from build123d import *

# Parameters (mm, degrees)
ESQUISSE2_W             = 8.320302529
ESQUISSE2_H             = 23.371875391
ESQUISSE2_W_2           = 7.922092332
ENL_V_MAT_EXTRU_1_DEPTH = 32
ENL_V_START             = -2
ENL_V_MAT_EXTRU_2_DEPTH = 2
ESQUISSE4_R             = 1
ENL_V_MAT_EXTRU_3_DEPTH = 4
ESQUISSE5_W             = 12.730996015
ESQUISSE5_H             = 15.162705394
ENL_V_MAT_EXTRU_4_DEPTH = 8


with BuildPart() as part:
    # Esquisse1 → Révolution1 (revolve)
    with BuildSketch(Plane.XY, mode=Mode.PRIVATE) as r_volution1_sk:
        Polygon((-14, 0), (-14, -2), (-3, -2), (-3, -4), (-2, -4), (-2, -7), (0, -7), (0, -11), (14.4, -11), (14.4, -10.25), (46.4, -10.25), (46.4, -3), (48.4, -3), (48.4, 0), align=None)
    revolve(r_volution1_sk.sketch.rotate(Axis((38.703399471, 0, 0), (-1, 0, 0)), 270), axis=Axis((38.703399471, 0, 0), (-1, 0, 0)))

    # Esquisse2 → Enlèv. mat.-Extru.1 (cut)
    with BuildSketch(Plane(origin=(46.4, 0, 0), x_dir=(0, 0, -1), z_dir=(1, 0, 0))):
        with Locations((-11.860151265, -0.490104857)):
            Rectangle(ESQUISSE2_W, ESQUISSE2_H)
        with Locations((11.661046166, -0.490104857)):
            Rectangle(ESQUISSE2_W_2, ESQUISSE2_H)
    extrude(amount=-ENL_V_MAT_EXTRU_1_DEPTH, mode=Mode.SUBTRACT)

    # Esquisse3 → Enlèv. mat.-Extru.2 (cut)
    with BuildSketch(Plane.ZY.offset(2).offset(ENL_V_START)):
        with BuildLine():
            Line((6.792150444, 1.69313093), (1.69313093, 6.792150444))
            ThreePointArc((1.69313093, 6.792150444), (4.949747468, 4.949747468), (6.792150444, 1.69313093))
        make_face()
        with BuildLine():
            Line((-6.792150444, -1.69313093), (-1.69313093, -6.792150444))
            ThreePointArc((-1.69313093, -6.792150444), (-4.949747468, -4.949747468), (-6.792150444, -1.69313093))
        make_face()
    extrude(amount=ENL_V_MAT_EXTRU_2_DEPTH, mode=Mode.SUBTRACT)

    # Esquisse4 → Enlèv. mat.-Extru.3 (cut)
    with BuildSketch(Plane.ZY):
        with Locations((0, 9)):
            Circle(ESQUISSE4_R)
        with Locations((-9, 0)):
            Circle(ESQUISSE4_R)
        with Locations((0, -9)):
            Circle(ESQUISSE4_R)
        with Locations((9, 0)):
            Circle(ESQUISSE4_R)
    extrude(amount=-ENL_V_MAT_EXTRU_3_DEPTH, mode=Mode.SUBTRACT)

    # Esquisse5 → Enlèv. mat.-Extru.4 (cut)
    with BuildSketch(Plane.ZY.offset(14)):
        with Locations((7.865498008, 1.780904513)):
            Rectangle(ESQUISSE5_W, ESQUISSE5_H)
    extrude(amount=-ENL_V_MAT_EXTRU_4_DEPTH, mode=Mode.SUBTRACT)


solid = part.part
Can you work these out from the model? Positions are in its coordinate system, mm. A direction names the side the tool comes from. Give positions to 0.01 mm unless a question says otherwise; leave off trailing zeros. Order: outer loops, then holes, each group sorted by start corner. A loop starts at its lowest first (then second) coordinate and runs counter-clockwise, first axis right, second up. Notation, with made-up numbers: M 12.25,-33.5 L 25.25,-33.5 A19 ccw 25.25,-24.5 Z; hole C -9.5,61 d6. An arc over 180 degrees is marked long. Use a Markdown table: item, result. Add a question column.
Item 1: We'd pull the mould along Z, two halves only. Please class faces 1 (the flat face through (4, 9, 0)), 2 (the flat face through (-14, 0, 0)), 3 (the flat face through (4, -9, 0)), 4 (the cylindrical face through (30.62, 10.25, 0.12)): +Z half, -Z half, draft (parallel to the pull), parting line (faces both ways), or undercut.
Item 2: Suppose I cut it at C-C (x = 44). List the corners of the cut face in (y, z) for me, then the cut area to 3 significant figures.
Item 3: For faces 5 (the flat face through (-0.986, -4.207, -4.278)), 6 (the cylindrical face through (30.62, -10.25, -0.12)), 7 (the flat face through (14.4, 0, -8)), 8 (the flat face through (-10, 0, 1.5)), 9 (the flat face through (4, 0, -9)), which set-ups out of +Z, -Z, +X, -X, +Y, -Y let a thin tool reach every point of the face, with its end or its side?
Item 4: Suppose I cut it at D-D (z = -9). List the corners of the cut face in (x, y) for me.
Item 5: If I drill on L1, parallel to Y at x = 2.6, z = 0; L2, parallel to Y at x = 32.5, z = -7.5; L3, parallel to Z at x = 23.5, y = -3, over which ranges is the centre line in solid material (lowest first)? Write a range as [from, to].
Item 6: Will these pins go through, and if not, where does the flat tip stop? pin 1 (10 mm diameter, centred on x = 35, y = 1.5, fed in from -Z); pin 2 (3 mm diameter, centred on y = 9, z = 0, fed in from -X); pin 3 (3 mm diameter, centred on x = 16, y = -3.5, fed in from +Z).
Answer sheet:
| question | item | result |
|---|---|---|
| 1 | face 1 | undercut |
| 1 | face 2 | draft |
| 1 | face 3 | undercut |
| 1 | face 4 | parting line |
| 2 | outline | M -6.77,-7.7 L 6.77,-7.7 A10.25 ccw 6.77,7.7 L -6.77,7.7 A10.25 ccw Z |
| 2 | area | 283 mm² |
| 3 | face 5 | -Z, -X, -Y |
| 3 | face 6 | +X, -Y |
| 3 | face 7 | +X |
| 3 | face 8 | +Z, -X, +Y, -Y |
| 3 | face 9 | -X |
| 4 | outline | M 0,-6.32 L 14.4,-6.32 L 14.4,6.32 L 0,6.32 L 0,1 L 4,1 L 4,-1 L 0,-1 Z |
| 5 | L1 | y = [-11, -10], [-8, 8], [10, 11] |
| 5 | L2 | y = [-6.99, 6.99] |
| 5 | L3 | z = [-7.7, 7.7] |
| 6 | pin 1 | stops at z = -7.7 |
| 6 | pin 2 | stops at x = 0 |
| 6 | pin 3 | stops at z = 7.7 |
